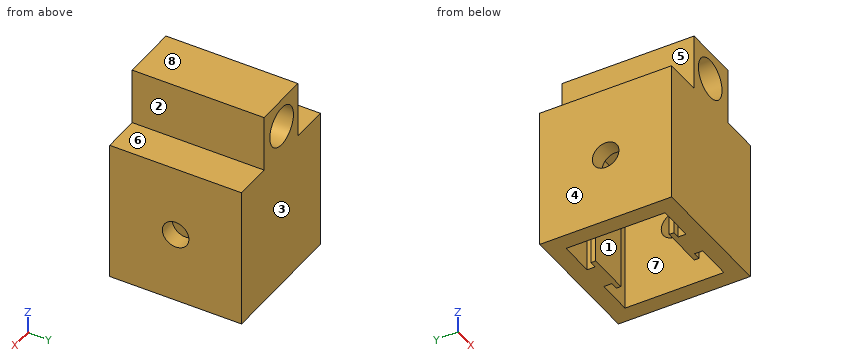
from build123d import *

# Parameters (mm, degrees)
EXTRUDE_2_DEPTH     = 30
EXTRUDE_2_2_DEPTH   = 30
EXTRUDE_3_DEPTH     = 5
SKETCH_2_5_W        = 28
SKETCH_2_5_H        = 28
SKETCH_2_5_W_2      = 21
SKETCH_2_5_H_2      = 21
EXTRUDE_4_DEPTH     = 30
CUT_EXTRUDE_1_DEPTH = 44.358966777
SKETCH_6_W          = 12
SKETCH_6_H          = 28
EXTRUDE_7_DEPTH     = 12
SKETCH_9_R          = 4.2
CUT_EXTRUDE_3_DEPTH = 44.358966777


with BuildPart() as part:
    # Sketch 2 → Extrude 2 (new body)
    with BuildSketch(Plane.XY):
        Polygon((-2.993279065, -10.5), (2.906720935, -10.5), (2.906720935, -8.8), (4.505554414, -8.8), (4.505554414, -7.799871607), (-4.495247842, -7.799871607), (-4.495247842, -8.8), (-2.993279065, -8.8), align=None)
    extrude(amount=-EXTRUDE_2_DEPTH)



with BuildPart() as body_2:
    # Sketch 2 → Extrude 2 2 (new body)
    with BuildSketch(Plane.XY):
        Polygon((2.906720935, 8.8), (2.906720935, 10.5), (-2.993279065, 10.5), (-2.993279065, 8.8), (-4.495247842, 8.8), (-4.495247842, 7.799871607), (4.505554414, 7.799871607), (4.505554414, 8.8), align=None)
    extrude(amount=-EXTRUDE_2_2_DEPTH)


with BuildPart() as part_1:
    add(part.part)

    add(body_2.part)  # Extrude 3 merges body 2
    # Sketch 2_4 → Extrude 3 (add)
    with BuildSketch(Plane.XY):
        Polygon((-10.5, 0), (10.5, 0), (10.5, 10.5), (2.906720935, 10.5), (2.906720935, 8.8), (4.505554414, 8.8), (4.505554414, 7.799871607), (-4.495247842, 7.799871607), (-4.495247842, 8.8), (-2.993279065, 8.8), (-2.993279065, 10.5), (-10.5, 10.5), align=None)
        Polygon((10.5, -10.5), (10.5, 0), (-10.5, 0), (-10.5, -10.5), (-2.993279065, -10.5), (-2.993279065, -8.8), (-4.495247842, -8.8), (-4.495247842, -7.799871607), (4.505554414, -7.799871607), (4.505554414, -8.8), (2.906720935, -8.8), (2.906720935, -10.5), align=None)
    extrude(amount=-EXTRUDE_3_DEPTH)

    # Sketch 2_5 → Extrude 4 (add)
    with BuildSketch(Plane.XY):
        Rectangle(SKETCH_2_5_W, SKETCH_2_5_H)
        Rectangle(SKETCH_2_5_W_2, SKETCH_2_5_H_2, mode=Mode.SUBTRACT)
    extrude(amount=-EXTRUDE_4_DEPTH)

    # Sketch 5 → Cut-Extrude 1 (cut, through all)
    with BuildSketch(Plane.ZY.offset(14)):
        with BuildLine():
            ThreePointArc((-17.82, 0), (-15, -2.82), (-12.18, 0))
            Line((-12.18, 0), (-17.82, 0))
        make_face()
        with BuildLine():
            Line((-17.82, 0), (-12.18, 0))
            ThreePointArc((-12.18, 0), (-15, 2.82), (-17.82, 0))
        make_face()
    extrude(amount=-CUT_EXTRUDE_1_DEPTH, mode=Mode.SUBTRACT)

    # Sketch 6 → Extrude 7 (add)
    with BuildSketch(Plane.XY):
        Rectangle(SKETCH_6_W, SKETCH_6_H)
    extrude(amount=EXTRUDE_7_DEPTH)

    # Sketch 9 → Cut-Extrude 3 (cut, through all)
    with BuildSketch(Plane.XZ.offset(14)):
        with Locations(Location((-0.251999231, 5.964564793, 0), (0, 0, 270))):
            Circle(SKETCH_9_R)
    extrude(amount=-CUT_EXTRUDE_3_DEPTH, mode=Mode.SUBTRACT)


solid = part_1.part
The listing builds one solid part. Answer for the finished solid, in the listing's coordinates (mm). Face numbers are marked on the shaded views. A direction names the side the tool comes from. Round coordinates to 2 decimals unless told otherwise and drop trailing zeros. Order: outer loops, then holes, each group sorted by start corner. A loop starts at its lowest first (then second) coordinate and runs counter-clockwise, first axis right, second up. Notation, with made-up numbers: (23, 81) -> (45, 81) arc R20 cw to (45, 100) -> close; hole circle Ø2 at (4, 88). An arc over 180 degrees is marked (long way). One line per item, written item: value.
Item 1: Find section D-D, the plane x = -6.75. Give the vertices of the cut face in (y, z).
Taken from the geometry:
outline: (-14, -30) -> (-10.5, -30) -> (-10.5, -5) -> (10.5, -5) -> (10.5, -30) -> (14, -30) -> (14, 0) -> (-14, 0) -> close
Item 2: Find section C-C, the plane y = -4.25. Give the vertices of the cut face in (x, z).
Taken from the geometry:
outline: (-14, -30) -> (-10.5, -30) -> (-10.5, -5) -> (10.5, -5) -> (10.5, -30) -> (14, -30) -> (14, 0) -> (6, 0) -> (6, 12) -> (-6, 12) -> (-6, 0) -> (-14, 0) -> close; hole circle Ø8.4 at (-0.25, 5.96)
Item 3: Straight lines are drawn through the part: L1, parallel to Y at x = -6.75, z = -14.5; L2, parallel to Y at x = 13.3, z = -15. For each, find the intervals that lie inside material, in ascending order.
Taken from the geometry:
L1: y = -14 to -10.5, 10.5 to 14
L2: y = -14 to -2.82, 2.82 to 14
Item 4: Find section A-A, the plane y = 0. Give the vertices of the cut face in (x, z).
Taken from the geometry:
outline: (-14, -30) -> (-10.5, -30) -> (-10.5, -17.82) -> (-14, -17.82) -> close; (-14, -12.18) -> (-10.5, -12.18) -> (-10.5, -5) -> (10.5, -5) -> (10.5, -12.18) -> (14, -12.18) -> (14, 0) -> (6, 0) -> (6, 12) -> (-6, 12) -> (-6, 0) -> (-14, 0) -> close; (10.5, -30) -> (14, -30) -> (14, -17.82) -> (10.5, -17.82) -> close; hole circle Ø8.4 at (-0.25, 5.96)
Item 5: Find section B-B, the plane z = -19. Give the vertices of the cut face in (x, y), then the cut area to 3 significant figures.
Taken from the geometry:
outline: (-14, -14) -> (14, -14) -> (14, 14) -> (-14, 14) -> close; hole (-10.5, -10.5) -> (-2.99, -10.5) -> (-2.99, -8.8) -> (-4.5, -8.8) -> (-4.5, -7.8) -> (4.51, -7.8) -> (4.51, -8.8) -> (2.91, -8.8) -> (2.91, -10.5) -> (10.5, -10.5) -> (10.5, 10.5) -> (2.91, 10.5) -> (2.91, 8.8) -> (4.51, 8.8) -> (4.51, 7.8) -> (-4.5, 7.8) -> (-4.5, 8.8) -> (-2.99, 8.8) -> (-2.99, 10.5) -> (-10.5, 10.5) -> close
area: 381 mm2
Item 6: Given P1, Ø3.5, axis at y = 6.5, z = 3, coming from the -X side; P2, Ø6.5, axis at y = 0, z = -15, coming from the +X side; P3, Ø5, axis at y = 9, z = 5.5, coming from the +X side, each flat-ended and moving along its own axis, determine where each tip first touches the part or whether it passes through.
Taken from the geometry:
P1: stops at x = -6
P2: stops at x = 14
P3: stops at x = 6
Item 7: For the marked faces 5, 6, 7 and 8, determine the directions among +Z, -Z, +X, -X, +Y, -Y from which every point of the face is accessible in a straight line to the end or side of a thin tool.
Taken from the geometry:
face 5: +Z, -X, +Y, -Y
face 6: +Z, +X, +Y, -Y
face 7: -Z
face 8: +Z, +X, -X, +Y, -Y
Item 8: For a pull along X with two mould halves and no side action, classify the marked faces 1, 2, 3 and 4 as released by +X, released by -X, zero draft, split by the parting line, or undercut.
Taken from the geometry:
face 1: undercut
face 2: released by +X
face 3: zero draft
face 4: released by -X
